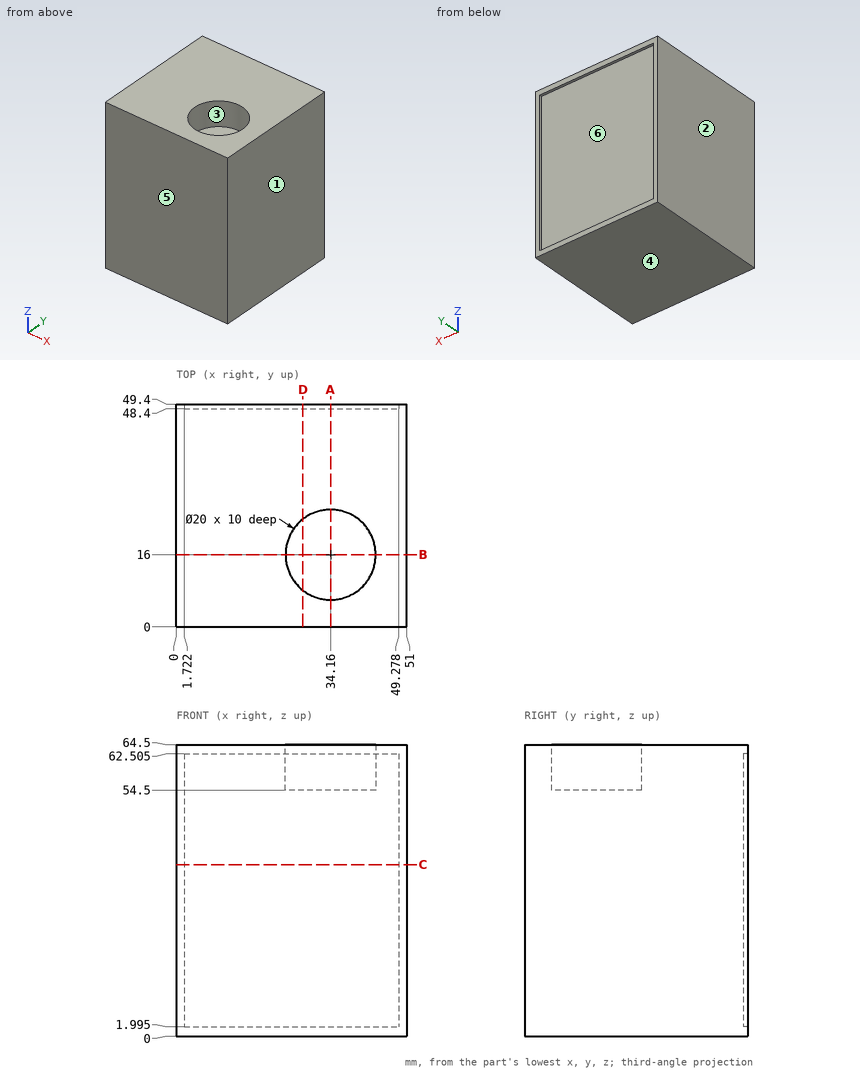
Answer from the drawing. Dimensions are ordinates in mm from the lowest x, y and z of the part. A direction names the side the tool comes from. Give positions to 0.01 mm unless a question says otherwise; leave off trailing zeros. Order: outer loops, then holes, each group sorted by start corner. A loop starts at its lowest first (then second) coordinate and runs counter-clockwise, first axis right, second up. Notation, with made-up numbers: (42, -24.5) -> (75, -24.5) arc R15 cw to (75, 4.5) -> close; hole circle Ø7 at (73.5, 32). An arc over 180 degrees is marked (long way). Answer as a JSON object with one key per item and string values. Group by question number.
1. Flat-ended cylindrical pins translate along their axes: pin 1 Ø14.5 at (x, z) = (15, 24) entering from +Y; pin 2 Ø18 at (x, y) = (34.16, 16) entering from +Z. Find the tip coordinate at first contact, or state that the pin passes through.
2. Section D-D on x = 28 is taken. Determine the outline of the cut face in (y, z) (1 decimal), plus the area to 3 significant figures.
3. A tool of negligible diameter and unlimited length cuts with its end or side. For the marked faces 5 and 6, from which of +Z, -Z, +X, -X, +Y, -Y can it reach the whole face along a straight path? Write none if from no direction.
4. Section B-B on y = 16 is taken. Determine the outline of the cut face in (x, z), plus the area to 3 significant figures.
5. Section A-A on x = 34.16 is taken. Determine the outline of the cut face in (y, z) (1 decimal), plus the area to 3 significant figures.
6. The mould has two halves that part along X. Classify the marked faces 1, 2, 3 and 4: released by +X, released by -X, zero draft, split by the parting line, or undercut.
7. Consider line 1 along Y through (x, z) = (34.16, 62.75); line 2 along Y through (x, z) = (32, 20); line 3 along Y through (x, z) = (34.16, 57). Determine where each line is inside the solid, lowest interval first. Write a range as [from, to].
8. Section C-C on z = 38 is taken. Determine the outline of the cut face in (x, y), plus the area to 3 significant figures.
Result sheet:
{
 "1": {"pin 1": "stops at y = 48.4", "pin 2": "stops at z = 54.5"},
 "2": {"outline": "(0, 0) -> (49.4, 0) -> (49.4, 2) -> (48.4, 2) -> (48.4, 62.5) -> (49.4, 62.5) -> (49.4, 64.5) -> (23.9, 64.5) -> (23.9, 54.5) -> (8.1, 54.5) -> (8.1, 64.5) -> (0, 64.5) -> close", "area": "2,970 mm^2"},
 "3": {"face 5": "+Z, -Z, +X, -X, -Y", "face 6": "+Y"},
 "4": {"outline": "(0, 0) -> (51, 0) -> (51, 64.5) -> (44.16, 64.5) -> (44.16, 54.5) -> (24.16, 54.5) -> (24.16, 64.5) -> (0, 64.5) -> close", "area": "3,090 mm^2"},
 "5": {"outline": "(0, 0) -> (49.4, 0) -> (49.4, 2) -> (48.4, 2) -> (48.4, 62.5) -> (49.4, 62.5) -> (49.4, 64.5) -> (26, 64.5) -> (26, 54.5) -> (6, 54.5) -> (6, 64.5) -> (0, 64.5) -> close", "area": "2,930 mm^2"},
 "6": {"face 1": "released by +X", "face 2": "released by -X", "face 3": "undercut", "face 4": "zero draft"},
 "7": {"line 1": "y = [0, 6], [26, 49.4]", "line 2": "y = [0, 48.4]", "line 3": "y = [0, 6], [26, 48.4]"},
 "8": {"outline": "(0, 0) -> (51, 0) -> (51, 49.4) -> (49.28, 49.4) -> (49.28, 48.4) -> (1.72, 48.4) -> (1.72, 49.4) -> (0, 49.4) -> close", "area": "2,470 mm^2"}
}
